Design review of the part built by this model. Coordinates are the model's own, in mm. A direction names the side the tool comes from. Coordinates: 2 decimals unless noted, no trailing zeros. Loops run counter-clockwise (first coordinate to the right, second up) from the corner with the lowest first, then second, coordinate; pieces in that order, holes last. Notation, with made-up numbers: (26, 32.25) -> (78, 32.25) arc R25 cw to (78, 54.25) -> close; hole circle Ø8 at (21.25, 29). An arc over 180 degrees is marked (long way). One line per item, written item: value. Start each with the question number.
1. Insertion check: pin 1 (3 mm diameter, centred on x = 14, y = 58.5, fed in from +Z); pin 2 (21.5 mm diameter, centred on x = 59.5, y = 53.5, fed in from -Z). Each pin has a flat end and moves straight along its axis. Give the tip position at first contact, or say it passes through.
2. Add section A-A on z = 263. Write out the cut boundary in (x, y).
3. Draft analysis for pull direction X (two halves, no side actions). For faces 5 (the flat face through (102.329, 63, 164)), 6 (the cylindrical face through (9.6, 64.35, 322.21)), 7 (the flat face through (85, 67, -6.35)), state which applies: pulls with the +X half, pulls with the -X half, needs draft (parallel to the pull), parting line crosses it, or undercut.
4. Machinability: for faces 1 (the flat face through (49, 124.5, 164)), 2 (the flat face through (48, 0, 164)), 3 (the cylindrical face through (101.096, 62.784, 294.993)), 4 (the cylindrical face through (88.7, 65.6, -3.1)), which of the approach directions +Z, -Z, +X, -X, +Y, -Y give a long, thin tool a straight path to every point of the face, cutting with its end or side? Answer none if there is none.
5. Add section C-C on y = 63.5. Write out the cut boundary in (x, z), plus the area to 3 significant figures.
6. Add section B-B on y = 44. Write out the cut boundary in (x, z), plus the area to 3 significant figures.
7. For probe 1 along Y at (x, z) = (51, 190); probe 2 along Z at (x, y) = (51.5, 50.5); probe 3 along X at (y, z) = (36, 131), list the stretches that pass through material, from the lowest coordinate up.
8. Add section D-D on x = 92.5. Write out the cut boundary in (y, z).
```python
from build123d import *

# Parameters (mm, degrees)
F0_W      = 102.32898
F0_H      = 127
F1_DEPTH  = 332.19898
F2_R      = 27.39898
F3_R      = 5.08
F5_T      = -2.5
F7_DEPTH  = 2.5
F4_R      = 5.50037
F8_DEPTH  = 2.5
F9_R      = 5.50037
F9_R_2    = 3.5
F10_DEPTH = 6.35
F11_DEPTH = 2.5


with BuildPart() as f1:
    # F0 (on Top) → F1 (new body)
    with BuildSketch(Plane.XY):
        with Locations((51.16449, 63.5)):
            Rectangle(F0_W, F0_H)
    extrude(amount=F1_DEPTH)

    # F2
    f2_edges = [f1.edges().sort_by_distance(p)[0] for p in [
        (0, 63.5, 332.19898),
    ]]
    fillet(f2_edges, radius=F2_R)

    # F3
    f3_edges = [f1.edges().sort_by_distance(p)[0] for p in [
        (102.32898, 0, 166.09949),
        (102.32898, 127, 166.09949),
    ]]
    fillet(f3_edges, radius=F3_R)

    # F5
    f5_openings = [f1.faces().sort_by_distance(p)[0] for p in [
        (51.121814, 63.5, 0),
    ]]
    offset(amount=F5_T, openings=f5_openings)

    # F6 (on face) → F7 (join)
    with BuildSketch(Plane(origin=(0, 0, 0), x_dir=(1, 0, 0), z_dir=(0, 0, -1))):
        with BuildLine():
            Line((102.32898, -121.92), (102.32898, -5.08))
            ThreePointArc((102.32898, -5.08), (100.8410824484, -1.4878975516), (97.24898, 0))
            Line((97.24898, 0), (0, 0))
            Line((0, 0), (0, -127))
            Line((0, -127), (97.24898, -127))
            ThreePointArc((97.24898, -127), (100.8410824484, -125.5121024484), (102.32898, -121.92))
        make_face()
    extrude(amount=-F7_DEPTH)

    # F4 (on face) → F8 (cut, through all)
    with BuildSketch(Plane.YZ.offset(102.32898)):
        with Locations((63.5, 289.53968)):
            Circle(F4_R)
    extrude(amount=-F8_DEPTH, mode=Mode.SUBTRACT)

    # F9 (on face) → F10 (join)
    with BuildSketch(Plane(origin=(0, 0, 0), x_dir=(1, 0, 0), z_dir=(0, 0, -1))):
        with Locations((83.6168, -63.5)):
            Circle(F9_R)
        with Locations((83.6168, -63.5)):
            Circle(F9_R_2, mode=Mode.SUBTRACT)
    extrude(amount=F10_DEPTH)

    # F11 (cut, through all): a face of the model
    f11_faces = [f1.faces().sort_by_distance(p)[0] for p in [
        (83.6168, 63.5, 0),
    ]]
    extrude(f11_faces, amount=-F11_DEPTH, mode=Mode.SUBTRACT)


solid = f1.part
```
Worked answers:
1. pin 1: stops at z = 329.48
1. pin 2: stops at z = 0
2. outline: (0, 0) -> (97.25, 0) arc R5.08 ccw to (102.33, 5.08) -> (102.33, 121.92) arc R5.08 ccw to (97.25, 127) -> (0, 127) -> close; hole (2.5, 2.5) -> (97.25, 2.5) arc R2.58 ccw to (99.83, 5.08) -> (99.83, 121.92) arc R2.58 ccw to (97.25, 124.5) -> (2.5, 124.5) -> close
3. face 5: pulls with the +X half
3. face 6: undercut
3. face 7: needs draft
4. face 1: none
4. face 2: +Z, -Z, +X, -X, -Y
4. face 3: +X
4. face 4: -Z
5. outline: (0, 0) -> (78.12, 0) -> (78.12, -6.35) -> (80.12, -6.35) -> (80.12, 2.5) -> (2.5, 2.5) -> (2.5, 304.8) arc R24.9 cw to (27.4, 329.7) -> (99.83, 329.7) -> (99.83, 295.04) -> (102.33, 295.04) -> (102.33, 332.2) -> (27.4, 332.2) arc R27.4 ccw to (0, 304.8) -> close; (87.12, -6.35) -> (89.12, -6.35) -> (89.12, 0) -> (102.33, 0) -> (102.33, 284.04) -> (99.83, 284.04) -> (99.83, 2.5) -> (87.12, 2.5) -> close
5. area: 2,100 mm²
6. outline: (0, 0) -> (102.33, 0) -> (102.33, 332.2) -> (27.4, 332.2) arc R27.4 ccw to (0, 304.8) -> close; hole (2.5, 2.5) -> (99.83, 2.5) -> (99.83, 329.7) -> (27.4, 329.7) arc R24.9 ccw to (2.5, 304.8) -> close
6. area: 2,120 mm²
7. probe 1: y = 0 to 2.5, 124.5 to 127
7. probe 2: z = 0 to 2.5, 329.7 to 332.2
7. probe 3: x = 0 to 2.5, 99.83 to 102.33
8. outline: (0, 0) -> (127, 0) -> (127, 332.2) -> (0, 332.2) -> close; hole (2.5, 2.5) -> (124.5, 2.5) -> (124.5, 329.7) -> (2.5, 329.7) -> close
